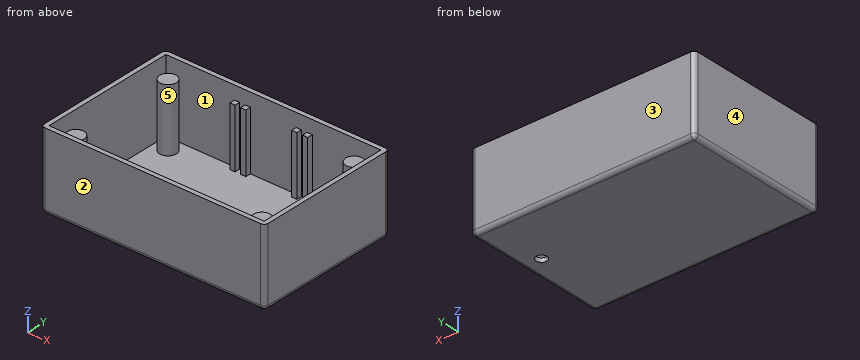
from build123d import *

# Parameters (mm, degrees)
CYLINDER040_R     = 2
CYLINDER040_DEPTH = 10
CYLINDER038_R     = 3.1
CYLINDER038_DEPTH = 23.5
BOX010_W          = 1.9
BOX010_H          = 2
BOX010_DEPTH      = 22
BOX009_W          = 79.7
BOX009_H          = 50.7
BOX009_DEPTH      = 27
BOX008_W          = 83
BOX008_H          = 54
BOX008_DEPTH      = 28.5
FILLET_R          = 1.5


with BuildPart() as led_hole:
    # Cylinder040 → Cylinder040 (new body)
    with BuildSketch(Plane(origin=(52, 18.01, -10), x_dir=(1, 0, 0), z_dir=(0, 0, 1))):
        Circle(CYLINDER040_R)
    extrude(amount=CYLINDER040_DEPTH)


with BuildPart() as lid_col:
    # Cylinder038 → Cylinder038 (new body)
    with BuildSketch(Plane(origin=(7, 7, 1.5), x_dir=(1, 0, 0), z_dir=(0, 0, 1))):
        Circle(CYLINDER038_R)
    extrude(amount=CYLINDER038_DEPTH)


with BuildPart() as lid_col001:
    # Clone010 base: copy of lid-col
    add(lid_col.part)


with BuildPart() as lid_col001_1:
    # Clone010 placement: moved
    add(lid_col001.part.moved(Location((0, 40, 0))))


with BuildPart() as lid_col002:
    # Clone011 base: copy of lid-col
    add(lid_col.part)


with BuildPart() as lid_col002_1:
    # Clone011 placement: moved
    add(lid_col002.part.moved(Location((69, 0, 0))))


with BuildPart() as lid_col003:
    # Clone012 base: copy of lid-col
    add(lid_col.part)


with BuildPart() as lid_col003_1:
    # Clone012 placement: moved
    add(lid_col003.part.moved(Location((69, 40, 0))))


with BuildPart() as lid_pin:
    # Box010 → Box010 (new body)
    with BuildSketch(Plane(origin=(50, 50.35, 1.5), x_dir=(1, 0, 0), z_dir=(0, 0, 1))):
        with Locations((0.95, 1)):
            Rectangle(BOX010_W, BOX010_H)
    extrude(amount=BOX010_DEPTH)


with BuildPart() as lid_pin001:
    # Clone003 base: copy of lid-pin
    add(lid_pin.part)


with BuildPart() as lid_pin001_1:
    # Clone003 placement: moved
    add(lid_pin001.part.moved(Location((4, 0, 0))))


with BuildPart() as lid_pin002:
    # Clone004 base: copy of lid-pin
    add(lid_pin.part)


with BuildPart() as lid_pin002_1:
    # Clone004 placement: moved
    add(lid_pin002.part.moved(Location((-18.9, 0, 0))))


with BuildPart() as lid_pin003:
    # Clone005 base: copy of lid-pin
    add(lid_pin.part)


with BuildPart() as lid_pin003_1:
    # Clone005 placement: moved
    add(lid_pin003.part.moved(Location((-22.9, 0, 0))))


with BuildPart() as lid_pin004:
    # Clone006 base: copy of lid-pin
    add(lid_pin.part)


with BuildPart() as lid_pin004_1:
    # Clone006 placement: moved
    add(lid_pin004.part.moved(Location((0, -48.7, 0))))


with BuildPart() as lid_pin005:
    # Clone007 base: copy of lid-pin
    add(lid_pin.part)


with BuildPart() as lid_pin005_1:
    # Clone007 placement: moved
    add(lid_pin005.part.moved(Location((4, -48.7, 0))))


with BuildPart() as lid_pin006:
    # Clone008 base: copy of lid-pin
    add(lid_pin.part)


with BuildPart() as lid_pin006_1:
    # Clone008 placement: moved
    add(lid_pin006.part.moved(Location((-18.9, -48.7, 0))))


with BuildPart() as lid_pin007:
    # Clone009 base: copy of lid-pin
    add(lid_pin.part)


with BuildPart() as lid_pin007_1:
    # Clone009 placement: moved
    add(lid_pin007.part.moved(Location((-22.9, -48.7, 0))))


with BuildPart() as cube009:
    # Box009 → Box009 (new body)
    with BuildSketch(Plane(origin=(1.65, 1.65, 1.5), x_dir=(1, 0, 0), z_dir=(0, 0, 1))):
        with Locations((39.85, 25.35)):
            Rectangle(BOX009_W, BOX009_H)
    extrude(amount=BOX009_DEPTH)


with BuildPart() as obj1:
    # Box008 → Box008 (new body)
    with BuildSketch(Plane.XY):
        with Locations((41.5, 27)):
            Rectangle(BOX008_W, BOX008_H)
    extrude(amount=BOX008_DEPTH)

    # Fillet
    fillet_edges = [obj1.edges().sort_by_distance(p)[0] for p in [
        (0, 0, 14.25),
        (0, 54, 14.25),
        (0, 27, 0),
        (83, 0, 14.25),
        (83, 54, 14.25),
        (83, 27, 0),
        (41.5, 0, 0),
        (41.5, 54, 0),
    ]]
    fillet(fillet_edges, radius=FILLET_R)

    # Cut005: cut Cube009
    add(cube009.part, mode=Mode.SUBTRACT)

    # Fusion002: union lid-pin
    add(lid_pin.part)

    # Fusion003: union lid-pin007
    add(lid_pin007_1.part)

    # Fusion004: union lid-pin006
    add(lid_pin006_1.part)

    # Fusion005: union lid-pin005
    add(lid_pin005_1.part)

    # Fusion006: union lid-pin004
    add(lid_pin004_1.part)

    # Fusion007: union lid-pin003
    add(lid_pin003_1.part)

    # Fusion008: union lid-pin002
    add(lid_pin002_1.part)

    # Fusion009: union lid-pin001
    add(lid_pin001_1.part)

    # Fusion010: union lid-col
    add(lid_col.part)

    # Fusion011: union lid-col003
    add(lid_col003_1.part)

    # Fusion012: union lid-col002
    add(lid_col002_1.part)

    # Fusion013: union lid-col001
    add(lid_col001_1.part)


with BuildPart() as obj1_1:
    # Fusion013 placement: moved
    add(obj1.part.moved(Location((-23.8, -13.7, -8.5))))

    # Cut007: cut led-hole
    add(led_hole.part, mode=Mode.SUBTRACT)


solid = obj1_1.part
Geometry: final body of the model. Coordinates: model frame, mm. Face numbers are marked on the shaded views. A direction names the side the tool comes from. Give positions to 0.01 mm unless a question says otherwise; leave off trailing zeros. Write each loop counter-clockwise with the first axis right and the second up, starting at its lowest first coordinate (ties: lowest second). Pieces come first, ordered by that corner, then holes. Notation, with made-up numbers: (81, 22.5) - (94, 22.5) arc R18 ccw to (94, 56.5) - close; hole circle Ø9 at (48.25, 47). An arc over 180 degrees is marked (long way). Return JSON: item names as keys, results as strings. Group by question number.
1) Section B-B on x = 52. Return the cut outline in (y, z).
2) Set-up query: the marked faces 1 and 2. Return all of +Z, -Z, +X, -X, +Y, -Y with unobstructed straight access to the full face (end or side cutting, diameter ignored); none if empty.
3) Line query: line 1 (X direction, y = 28.5, z = 0.75); line 2 (X direction, y = 38, z = 5.5); line 3 (Y direction, x = -10.5, z = 9.5). Output: solid intervals per line, ascending.
4) Section D-D on y = -6.7. Return the cut outline in (x, z), plus the area to 3 significant figures.
5) Mould query, pull axis Y, two halves, no side actions, for the marked faces 3, 4 and 5. Classes: released by +Y, released by -Y, zero draft, split by the parting line, or undercut.
6) Section A-A on y = 18.01. Return the cut outline in (x, z), plus the area to 3 significant figures.
7) Section C-C on z = 1. State how many separate pieces and enclosed holes the cut face has, plus the area to 3 significant figures.
8) First-contact query: P1, Ø2, axis at x = 34.5, y = 5, coming from the +Z side; P2, Ø2, axis at x = 31, y = -11, coming from the +Z side; P3, Ø1.9, axis at x = 52.5, y = 32, coming from the +Z side. Flat tips, straight axial feed; report the tip coordinate or a pass-through.
Filled in:
{
 "1": {"outline": "(-13.7, -7) arc R1.5 ccw to (-12.2, -8.5) - (16.01, -8.5) - (16.01, -7) - (-3.61, -7) - (-3.61, 16.5) - (-9.79, 16.5) - (-9.79, -7) - (-12.05, -7) - (-12.05, 20) - (-13.7, 20) - close; (20.01, -8.5) - (38.8, -8.5) arc R1.5 ccw to (40.3, -7) - (40.3, 20) - (38.65, 20) - (38.65, -7) - (36.39, -7) - (36.39, 16.5) - (30.21, 16.5) - (30.21, -7) - (20.01, -7) - close"},
 "2": {"face 1": "+Z", "face 2": "+Z, -Z, +X, -X, -Y"},
 "3": {"line 1": "x = -23.8 to -22.15, 57.55 to 59.2", "line 2": "x = -23.8 to -22.15, 3.3 to 5.2, 7.3 to 9.2, 26.2 to 28.1, 30.2 to 32.1, 57.55 to 59.2", "line 3": "y = -13.7 to -12.05, 38.65 to 40.3"},
 "4": {"outline": "(-23.8, -7) arc R1.5 ccw to (-22.3, -8.5) - (57.7, -8.5) arc R1.5 ccw to (59.2, -7) - (59.2, 20) - (57.55, 20) - (57.55, -7) - (55.3, -7) - (55.3, 16.5) - (49.1, 16.5) - (49.1, -7) - (-13.7, -7) - (-13.7, 16.5) - (-19.9, 16.5) - (-19.9, -7) - (-22.15, -7) - (-22.15, 20) - (-23.8, 20) - close", "area": "504 mm^2"},
 "5": {"face 3": "released by +Y", "face 4": "zero draft", "face 5": "undercut"},
 "6": {"outline": "(-23.8, -7) arc R1.5 ccw to (-22.3, -8.5) - (50, -8.5) - (50, -7) - (-22.15, -7) - (-22.15, 20) - (-23.8, 20) - close; (54, -8.5) - (57.7, -8.5) arc R1.5 ccw to (59.2, -7) - (59.2, 20) - (57.55, 20) - (57.55, -7) - (54, -7) - close", "area": "207 mm^2"},
 "7": {"separate pieces": "5", "enclosed holes": "1", "area": "590 mm^2"},
 "8": {"P1": "stops at z = -7", "P2": "stops at z = 15", "P3": "stops at z = 16.5"}
}
